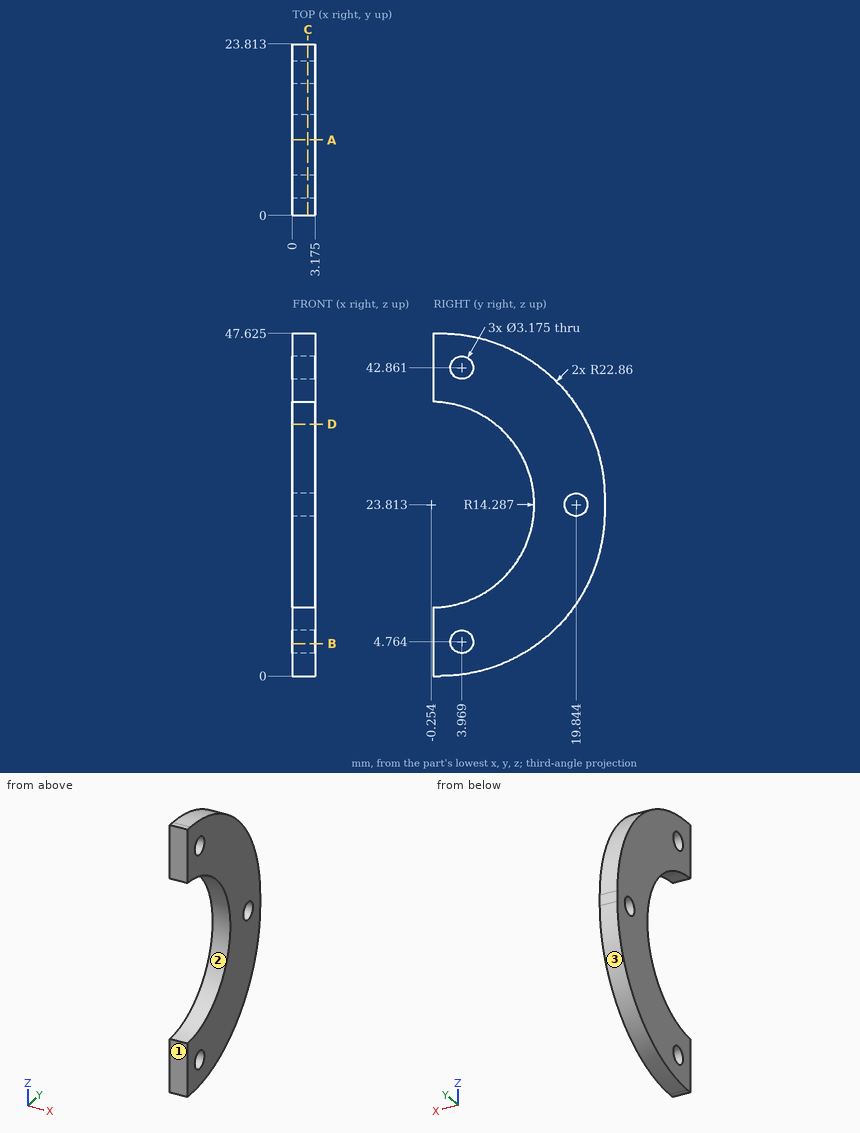
For this review, use the dimensioned drawing (mm, ordinates from the lowest corner) and the shaded views. Give positions to 0.01 mm unless a question says otherwise; leave off trailing zeros. Order: outer loops, then holes, each group sorted by start corner. A loop starts at its lowest first (then second) coordinate and runs counter-clockwise, first axis right, second up. Notation, with made-up numbers: M 23,85.5 L 29,85.5 A16 cw 29,90.5 Z; hole C 65,74 d10. An arc over 180 degrees is marked long. Use one line per item in the form item = value. Start each with the question number.
Item 1: We need section D-D on z = 35. Give the boundary of the cut face in (x, y) (1 decimal), plus the area to 3 significant figures.
Item 2: Insertion check: pin 1 Ø1.5 at (x, z) = (1, 22.5) entering from -Y; pin 2 Ø1 at (x, z) = (0.5, 25) entering from +Y. Each pin has a flat end and moves straight along its axis. Give the tip position at first contact, or say it passes through.
Item 3: We need section A-A on y = 10.5. Give the boundary of the cut face in (x, z) (1 decimal).
Item 4: We need section B-B on z = 4.5. Give the boundary of the cut face in (x, y) (1 decimal).
Item 5: We need section C-C on x = 2.15. Give the boundary of the cut face in (y, z) (1 decimal).
Item 6: The part is to be moulded in two halves that separate along Z. For the marked faces 1, 2 and 3, say which applies: pulls with the +Z half, pulls with the -Z half, needs draft (parallel to the pull), parting line crosses it, or undercut.
Item 7: To check wall thickness, follow line 1 along Z through (x, y) = (0.7, 5) (1 decimal); line 2 along Z through (x, y) = (1.5, 6.25) (1 decimal); line 3 along Z through (x, y) = (1.45, 10) (1 decimal). State the ranges of each line that lie inside material, in increasing order. Write a range as from..to.
Completed:
q1.outline = M 0,8.6 L 3.2,8.6 L 3.2,21.4 L 0,21.4 Z
q1.area = 40.5 mm²
q2.pin_1 = 13.88
q2.pin_2 = 23.81
q3.outline = M 0,2.1 L 3.2,2.1 L 3.2,14.4 L 0,14.4 Z; M 0,33.2 L 3.2,33.2 L 3.2,45.5 L 0,45.5 Z
q4.outline = M 0,0 L 3.2,0 L 3.2,2.4 L 0,2.4 Z; M 0,5.5 L 3.2,5.5 L 3.2,14.6 L 0,14.6 Z
q5.outline = M 0,0 L 1,0 A22.9 ccw 23.8,22.9 L 23.8,24.8 A22.9 ccw 1,47.6 L 0,47.6 L 0,38.1 A14.3 cw 0,9.5 Z; hole C 4,4.8 d3.2; hole C 4,42.9 d3.2; hole C 19.8,23.8 d3.2
q6.face_1 = needs draft
q6.face_2 = undercut
q6.face_3 = pulls with the -Z half
q7.line_1 = 0.4..3.6, 6..10.5, 37.1..41.7, 44.1..47.3
q7.line_2 = 0.6..11.1, 36.5..47
q7.line_3 = 1.9..13.9, 33.8..45.8
